from build123d import *

# Parameters (mm, degrees)
SKIZZE1_R                       = 2.45
AUFSATZ_LINEAR_AUSTRAGEN1_DEPTH = 1
AUFSATZ_LINEAR_AUSTRAGEN2_DEPTH = 0.4
VERRUNDUNG1_R                   = 0.5


with BuildPart() as part:
    # Skizze1 → Aufsatz-Linear austragen1 (new body)
    with BuildSketch(Plane.XY):
        Circle(SKIZZE1_R)
    extrude(amount=AUFSATZ_LINEAR_AUSTRAGEN1_DEPTH)

    # Skizze2 → Aufsatz-Linear austragen2 (add)
    with BuildSketch(Plane(origin=(0, 0, 0), x_dir=(-1, 0, 0), z_dir=(0, 0, -1))):
        with BuildLine():
            Line((-4.9, 2.65), (4.9, 2.65))
            ThreePointArc((4.9, 2.65), (7.55, 0), (4.9, -2.65))
            Line((4.9, -2.65), (-4.9, -2.65))
            ThreePointArc((-4.9, -2.65), (-7.55, 0), (-4.9, 2.65))
        make_face()
    extrude(amount=AUFSATZ_LINEAR_AUSTRAGEN2_DEPTH)

    # Verrundung1
    verrundung1_edges = [part.edges().sort_by_distance(p)[0] for p in [
        (-2.45, 0, 1),
    ]]
    fillet(verrundung1_edges, radius=VERRUNDUNG1_R)


solid = part.part
Could you check a few things on this model? Use its own coordinates, in mm. A direction names the side the tool comes from. Give positions to 0.01 mm unless a question says otherwise; leave off trailing zeros. Write each loop counter-clockwise with the first axis right and the second up, starting at its lowest first coordinate (ties: lowest second). Pieces come first, ordered by that corner, then holes. Notation, with made-up numbers: (28, -30.5) -> (41, -30.5) arc R14 ccw to (41, -25.5) -> close; hole circle Ø7 at (52.5, -14.5). An arc over 180 degrees is marked (long way). Write each question's results on one line, items separated by ' | '. Start each with the question number.
Q1. Suppose I cut it at B-B, the plane x = 0. List the corners of the cut face in (y, z) for me.
Q2. Suppose I cut it at D-D, the plane x = -3. List the corners of the cut face in (y, z) for me, and give its area (3 significant figures).
Q3. Which directions (+Z, -Z, +X, -X, +Y, -Y) give clear straight access to the entire face, cutting with the end or side of a thin tool? Please do faces 1 (the face through (7.55, -0.06, -0.2)), 2 (the face through (-0.5, -2.4, 0.2)).
Q4. Suppose I cut it at C-C, the plane z = -0.25. List the corners of the cut face in (x, y) for me.
Q5. Suppose I cut it at A-A, the plane y = 0. List the corners of the cut face in (x, z) for me, and give its area (3 significant figures).
Q6. I need wall thicknesses on probe 1 along Z at (x, y) = (6.25, 0.7); probe 2 along X at (y, z) = (-0.8, 0.75); probe 3 along X at (y, z) = (-1.3, 0.4). Which ranges of each line are inside material? Lowest first, please.
Outcome:
1) outline: (-2.65, -0.4) -> (2.65, -0.4) -> (2.65, 0) -> (2.45, 0) -> (2.45, 0.5) arc R0.5 ccw to (1.95, 1) -> (-1.95, 1) arc R0.5 ccw to (-2.45, 0.5) -> (-2.45, 0) -> (-2.65, 0) -> close
2) outline: (-2.65, -0.4) -> (2.65, -0.4) -> (2.65, 0) -> (-2.65, 0) -> close | area: 2.12 mm2
3) face 1: +Z, -Z, +X | face 2: +Z
4) outline: (-4.9, -2.65) -> (4.9, -2.65) arc R2.65 ccw to (4.9, 2.65) -> (-4.9, 2.65) arc R2.65 ccw to start
5) outline: (-7.55, -0.4) -> (7.55, -0.4) -> (7.55, 0) -> (2.45, 0) -> (2.45, 0.5) arc R0.5 ccw to (1.95, 1) -> (-1.95, 1) arc R0.5 ccw to (-2.45, 0.5) -> (-2.45, 0) -> (-7.55, 0) -> close | area: 10.8 mm2
6) probe 1: -0.4 to 0 | probe 2: -2.24 to 2.24 | probe 3: -2.08 to 2.08
